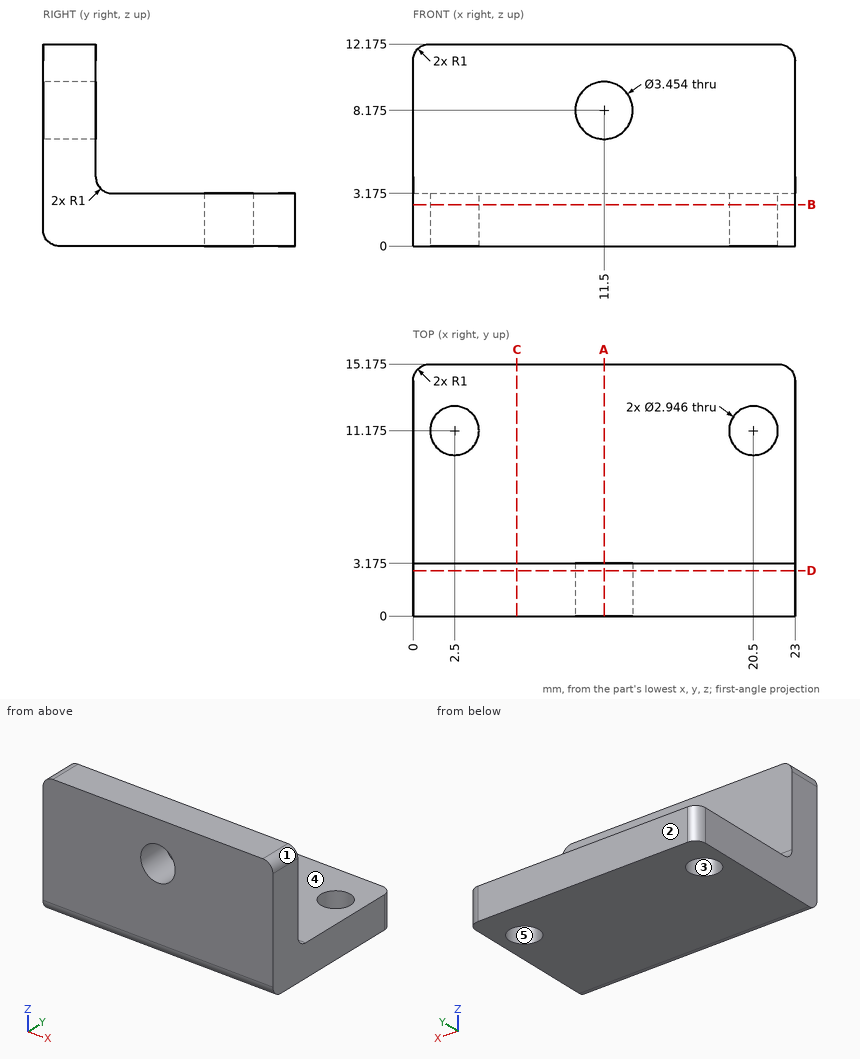
Drawing for the job (mm, zero at the part's lowest x, y, z). A direction names the side the tool comes from. Round coordinates to 2 decimals unless told otherwise and drop trailing zeros. Loops run counter-clockwise (first coordinate to the right, second up) from the corner with the lowest first, then second, coordinate; pieces in that order, holes last. Notation, with made-up numbers: (-1.5, 38) -> (44.5, 38) arc R18 cw to (44.5, 68) -> close; hole circle Ø10 at (-9, 0.25). An arc over 180 degrees is marked (long way). Answer as CSV lines item,"result". Start each with the question number.
1) Slice it at C-C (x = 6.25). List the corners of the cut face in (y, z) (1 decimal).
2) Pin check, flat tips, straight feed: P1, Ø6, axis at x = 18, z = 10, coming from the -Y side; P2, Ø2, axis at x = 8.5, z = 7.5, coming from the +Y side (3 decimals). Stop position of each tip, or through.
3) Slice it at D-D (y = 2.75). List the corners of the cut face in (x, z) (1 decimal), plus the area to 3 significant figures.
4) Mould opens along Y. For the marked faces 1, 2 and 3 say: +Y half, -Y half, draft (parallel to the pull), parting line (faces both ways), or undercut.
5) Slice it at A-A (x = 11.5). List the corners of the cut face in (y, z) (1 decimal).
6) Tool access for the marked faces 4 and 5: list every direction of +Z, -Z, +X, -X, +Y, -Y with a clear straight run to the whole face (end or side of a thin tool).
7) Probe line 1 along Z through (x, y) = (11.5, 1.05) (1 decimal); line 2 along Y through (x, z) = (20.5, 1.75) (1 decimal); line 3 along Z through (x, y) = (3.25, 9.75) (1 decimal). List the from-to ranges inside material, lowest first.
8) Slice it at B-B (z = 2.5). List the corners of the cut face in (x, y) (1 decimal).
Filled in:
1,outline,"(0, 1) arc R1 ccw to (1, 0) -> (15.2, 0) -> (15.2, 3.2) -> (4.2, 3.2) arc R1 cw to (3.2, 4.2) -> (3.2, 12.2) -> (0, 12.2) -> close"
2,P1,"stops at y = 0"
2,P2,"stops at y = 3.175"
3,outline,"(0, 0) -> (23, 0) -> (23, 11.2) arc R1 ccw to (22, 12.2) -> (1, 12.2) arc R1 ccw to (0, 11.2) -> close; hole circle Ø3.5 at (11.5, 8.2)"
3,area,"270 mm2"
4,face 1,"draft"
4,face 2,"+Y half"
4,face 3,"undercut"
5,outline,"(0, 1) arc R1 ccw to (1, 0) -> (15.2, 0) -> (15.2, 3.2) -> (4.2, 3.2) arc R1 cw to (3.2, 4.2) -> (3.2, 6.4) -> (0, 6.4) -> close; (0, 9.9) -> (3.2, 9.9) -> (3.2, 12.2) -> (0, 12.2) -> close"
6,face 4,"+Z, +X, -X, +Y"
6,face 5,"+Z, -Z"
7,line 1,"z = 0 to 6.4, 9.9 to 12.2"
7,line 2,"y = 0 to 9.7, 12.6 to 15.2"
7,line 3,"z = 0 to 3.2"
8,outline,"(0, 0) -> (23, 0) -> (23, 14.2) arc R1 ccw to (22, 15.2) -> (1, 15.2) arc R1 ccw to (0, 14.2) -> close; hole circle Ø2.9 at (2.5, 11.2); hole circle Ø2.9 at (20.5, 11.2)"
